Job drawing, mm, ordinate dimensions from the low corner. One solid piece. Coordinates: 2 decimals unless noted, no trailing zeros. Write each loop counter-clockwise with the first axis right and the second up, starting at its lowest first coordinate (ties: lowest second). Pieces come first, ordered by that corner, then holes. Notation, with made-up numbers: (76.5, 52) - (96.5, 52) arc R30 ccw to (96.5, 86) - close; hole circle Ø7 at (8.5, 71.5). An arc over 180 degrees is marked (long way). Use a Markdown table: item, result.
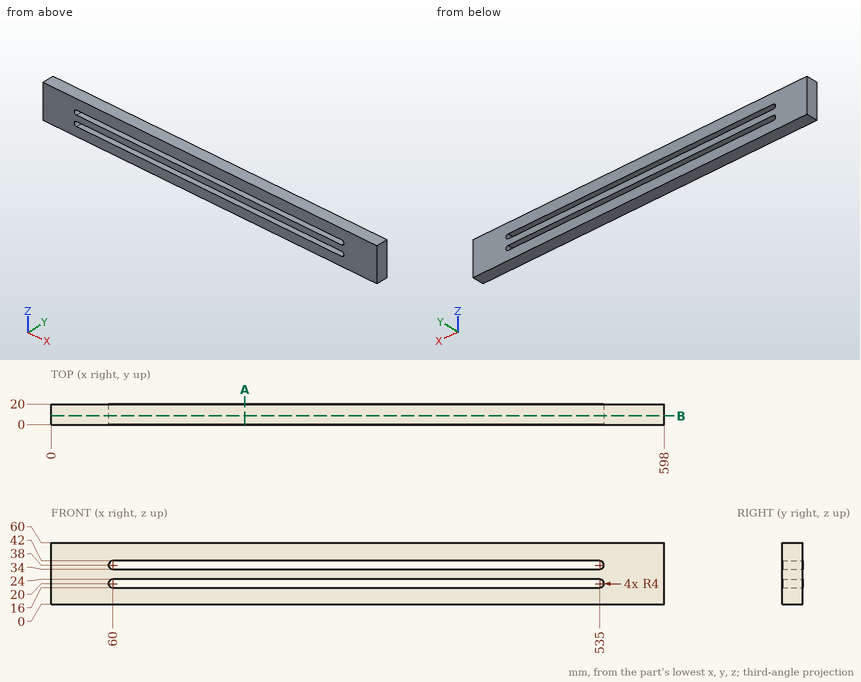
Item 1: Drill centre lines: probe 1 along Z at (x, y) = (193, 3); probe 2 along X at (y, z) = (17.75, 19.5); probe 3 along X at (y, z) = (11.5, 19). Where is each one in solid material? Low to high.
From the geometry:
| item | result |
|---|---|
| probe 1 | 0 to 16, 24 to 34, 42 to 60 |
| probe 2 | 0 to 56.03, 538.97 to 598 |
| probe 3 | 0 to 56.13, 538.87 to 598 |
Item 2: Band-saw the part on B-B, the plane y = 8.5. Give the cut face in (x, z), then the cut area to 3 significant figures.
From the geometry:
| item | result |
|---|---|
| outline | (0, 0) - (598, 0) - (598, 60) - (0, 60) - close; hole (60, 16) - (535, 16) arc R4 ccw to (535, 24) - (60, 24) arc R4 ccw to start; hole (60, 34) - (535, 34) arc R4 ccw to (535, 42) - (60, 42) arc R4 ccw to start |
| area | 28,200 mm^2 |
Item 3: Band-saw the part on A-A, the plane x = 189. Give the cut face in (y, z).
From the geometry:
| item | result |
|---|---|
| outline | (0, 0) - (20, 0) - (20, 16) - (0, 16) - close; (0, 24) - (20, 24) - (20, 34) - (0, 34) - close; (0, 42) - (20, 42) - (20, 60) - (0, 60) - close |
